Input: part model. Units: mm. Frame: model coordinates. A direction names the side the tool comes from. Round coordinates to 2 decimals unless told otherwise and drop trailing zeros. Loops run counter-clockwise (first coordinate to the right, second up) from the corner with the lowest first, then second, coordinate; pieces in that order, holes last. Notation, with made-up numbers: (81, 72) -> (135, 72) arc R10 cw to (135, 90) -> close; hole circle Ø7 at (-12.75, -25). An arc over 180 degrees is marked (long way). One line per question, with ' | ' between items. Start each with the question number.
Q1. Cut plane B-B on x = 3.5. Return loops of the section in (y, z).
Q2. Access query for faces 1 (the face through (22, 70, -15)), 2 (the face through (-8.14, 69.25, -46.06)). Directions: +Z, -Z, +X, -X, +Y, -Y. A direction counts if a zero-diameter tool reaches every point of the face in a straight line with its end or side. Return the directions, or none.
Q3. Contact query for flat-ended pins moving along their axis: P1, Ø8, axis at x = -9, y = 36, coming from the +Z side; P2, Ø2.5, axis at y = 71, z = -15, coming from the -X side; P3, Ø10, axis at y = 75.5, z = -7.5, coming from the -X side; P4, Ø10, axis at x = -20, y = 36, coming from the -Z side. Output: stop coordinate, or through.
Q4. Mould query, pull axis X, two halves, no side actions, for faces 3 (the face through (23, 54, -25)), 4 (the face through (21.028, 53.072, -3.464)), 5 (the face through (6.58, 65.9, -46.06)). Classes: pulls with the +X half, pulls with the -X half, needs draft (parallel to the pull), parting line crosses it, or undercut.
Q5. Cut plane C-C on y = 13.75. Return loops of the section in (x, z), and give its area (3 significant figures).
Q6. Cut plane D-D on z = -43.5. Return loops of the section in (x, y), and give its area (3 significant figures).
Q7. Material intervals for L1, parallel to Y at x = 22.7, z = -30.75; L2, parallel to Z at x = 22.6, y = 71; L3, parallel to Y at x = 22, z = -12, sorted ascending.
Q8. Cut plane A-A on z = -12. State how many separate pieces and enclosed holes the cut face has, and give its area (3 significant figures).
from build123d import *

# Parameters (mm, degrees)
BOSS_EXTRUDE1_DEPTH = 90
SKETCH2_R           = 10.1
CUT_EXTRUDE1_DEPTH  = 2.8
SKETCH3_R           = 2.5
SKETCH3_R_2         = 1
CUT_EXTRUDE2_DEPTH  = 22
SKETCH4_R           = 10.1
CUT_EXTRUDE3_DEPTH  = 10
FILLET1_R           = 10
CUT_EXTRUDE9_DEPTH  = 70
FILLET2_R           = 30
SKETCH9_R           = 2.5
SKETCH9_R_2         = 1
CUT_EXTRUDE11_DEPTH = 22.8
SKETCH10_R          = 10.1
CUT_EXTRUDE12_DEPTH = 2.8
SKETCH11_R          = 10.1
CUT_EXTRUDE13_DEPTH = 12.8
FILLET4_R           = 10
SKETCH13_W          = 1
SKETCH13_H          = 35
CUT_EXTRUDE14_DEPTH = 50
CUT_EXTRUDE20_DEPTH = 20


with BuildPart() as part:
    # Sketch1 → Boss-Extrude1 (new body)
    with BuildSketch(Plane(origin=(0, 0, 0), x_dir=(1, 0, 0), z_dir=(0, 1, 0))):
        Polygon((-27.5, 0), (-27.5, 42), (19, 42), (19, 0), (23, 0), (23, 50), (-30.5, 50), (-30.5, 0), align=None)
    extrude(amount=BOSS_EXTRUDE1_DEPTH)

    # Sketch2 → Cut-Extrude1 (cut)
    with BuildSketch(Plane.ZY.offset(-19)):
        with Locations((-12, 78)):
            Circle(SKETCH2_R)
    extrude(amount=-CUT_EXTRUDE1_DEPTH, mode=Mode.SUBTRACT)

    # Sketch3 → Cut-Extrude2 (cut)
    with BuildSketch(Plane.ZY.offset(-21.8)):
        with Locations((-12, 78)):
            Circle(SKETCH3_R)
        with Locations((-15, 85)):
            Circle(SKETCH3_R_2)
        with Locations((-12, 85)):
            Circle(SKETCH3_R_2)
        with Locations((-9, 85)):
            Circle(SKETCH3_R_2)
        with Locations((-19, 81)):
            Circle(SKETCH3_R_2)
        with Locations((-19, 78)):
            Circle(SKETCH3_R_2)
        with Locations((-19, 75)):
            Circle(SKETCH3_R_2)
        with Locations((-15, 71)):
            Circle(SKETCH3_R_2)
        with Locations((-12, 71)):
            Circle(SKETCH3_R_2)
        with Locations((-9, 71)):
            Circle(SKETCH3_R_2)
        with Locations((-5, 75)):
            Circle(SKETCH3_R_2)
        with Locations((-5, 78)):
            Circle(SKETCH3_R_2)
        with Locations((-5, 81)):
            Circle(SKETCH3_R_2)
    extrude(amount=-CUT_EXTRUDE2_DEPTH, mode=Mode.SUBTRACT)

    # Sketch4 → Cut-Extrude3 (cut)
    with BuildSketch(Plane.ZY.offset(30.5)):
        with Locations((-12, 78)):
            Circle(SKETCH4_R)
    extrude(amount=-CUT_EXTRUDE3_DEPTH, mode=Mode.SUBTRACT)

    # Fillet1
    fillet1_edges = [part.edges().sort_by_distance(p)[0] for p in [
        (21, 90, 0),
        (-29, 90, 0),
    ]]
    fillet(fillet1_edges, radius=FILLET1_R)

    # Sketch8 → Cut-Extrude9 (cut)
    with BuildSketch(Plane(origin=(23, 0, 0), x_dir=(0, 0, -1), z_dir=(1, 0, 0))):
        Polygon((0, 0), (10, 0), (10, 40), (0, 60), align=None)
        with BuildLine():
            Line((50, 45), (49.384007447, 45))
            ThreePointArc((49.384007447, 45), (46.548633561, 44.118331571), (44.713203531, 41.784261971))
            ThreePointArc((44.713203531, 41.784261971), (39.074197476, 21.242984276), (37.5, 0))
            Line((37.5, 0), (50, 0))
            Line((50, 0), (50, 45))
        make_face()
    extrude(amount=-CUT_EXTRUDE9_DEPTH, mode=Mode.SUBTRACT)

    # Fillet2
    fillet2_edges = [part.edges().sort_by_distance(p)[0] for p in [
        (-29, 40, -10),
        (21, 40, -10),
    ]]
    fillet(fillet2_edges, radius=FILLET2_R)

    # Sketch9 → Cut-Extrude11 (cut)
    with BuildSketch(Plane.ZY.offset(-19)):
        with Locations((-23.75, 13.75)):
            Circle(SKETCH9_R)
        with Locations((-23.75, 20.75)):
            Circle(SKETCH9_R_2)
        with Locations((-26.75, 20.75)):
            Circle(SKETCH9_R_2)
        with Locations((-20.75, 20.75)):
            Circle(SKETCH9_R_2)
        with Locations((-16.75, 10.75)):
            Circle(SKETCH9_R_2)
        with Locations((-16.75, 13.75)):
            Circle(SKETCH9_R_2)
        with Locations((-16.75, 16.75)):
            Circle(SKETCH9_R_2)
        with Locations((-26.75, 6.75)):
            Circle(SKETCH9_R_2)
        with Locations((-23.75, 6.75)):
            Circle(SKETCH9_R_2)
        with Locations((-20.75, 6.75)):
            Circle(SKETCH9_R_2)
        with Locations((-30.75, 16.75)):
            Circle(SKETCH9_R_2)
        with Locations((-30.75, 13.75)):
            Circle(SKETCH9_R_2)
        with Locations((-30.75, 10.75)):
            Circle(SKETCH9_R_2)
    extrude(amount=-CUT_EXTRUDE11_DEPTH, mode=Mode.SUBTRACT)

    # Sketch10 → Cut-Extrude12 (cut)
    with BuildSketch(Plane.ZY.offset(-19)):
        with Locations((-23.75, 13.75)):
            Circle(SKETCH10_R)
    extrude(amount=-CUT_EXTRUDE12_DEPTH, mode=Mode.SUBTRACT)

    # Sketch11 → Cut-Extrude13 (cut)
    with BuildSketch(Plane.ZY.offset(30.5)):
        with Locations((-23.75, 13.75)):
            Circle(SKETCH11_R)
    extrude(amount=-CUT_EXTRUDE13_DEPTH, mode=Mode.SUBTRACT)

    # Fillet4
    fillet4_edges = [part.edges().sort_by_distance(p)[0] for p in [
        (-29, 0, -10),
        (21, 0, -10),
        (21, 0, -37.5),
        (-29, 0, -37.5),
    ]]
    fillet(fillet4_edges, radius=FILLET4_R)

    # Sketch13 → Cut-Extrude14 (cut)
    with BuildSketch(Plane.XY):
        with Locations((-28, 17.5)):
            Rectangle(SKETCH13_W, SKETCH13_H)
    extrude(amount=-CUT_EXTRUDE14_DEPTH, mode=Mode.SUBTRACT)

    # Sketch14 → Cut-Extrude20 (cut)
    with BuildSketch(Plane(origin=(0, 0, -50), x_dir=(-1, 0, 0), z_dir=(0, 0, -1))):
        with BuildLine():
            Line((3.27778227, 69.250932504), (2.845176463, 68.801688012))
            ThreePointArc((2.845176463, 68.801688012), (0.391852409, 70.892666632), (-2.246261107, 72.745056327))
            ThreePointArc((-2.246261107, 72.745056327), (-6.625047437, 65.79780173), (-8.487956293, 57.799821563))
            ThreePointArc((-8.487956293, 57.799821563), (-5.961417112, 64.793099841), (-1.768021606, 70.933521279))
            ThreePointArc((-1.768021606, 70.933521279), (0.045073944, 69.272193574), (1.971595392, 67.743847957))
            ThreePointArc((1.971595392, 67.743847957), (-1.648113464, 59.360569649), (-0.654011446, 50.283488148))
            ThreePointArc((-0.654011446, 50.283488148), (-0.301953995, 59.840560068), (4.104319798, 68.328570399))
            ThreePointArc((4.104319798, 68.328570399), (8.510593592, 59.840560068), (8.862651043, 50.283488148))
            ThreePointArc((8.862651043, 50.283488148), (9.856753061, 59.360569649), (6.237044205, 67.743847957))
            ThreePointArc((6.237044205, 67.743847957), (8.163565653, 69.272193574), (9.976661203, 70.933521279))
            ThreePointArc((9.976661203, 70.933521279), (14.170056709, 64.793099841), (16.69659589, 57.799821563))
            ThreePointArc((16.69659589, 57.799821563), (14.833687034, 65.79780173), (10.454900704, 72.745056327))
            ThreePointArc((10.454900704, 72.745056327), (7.816787188, 70.892666632), (5.363463133, 68.801688012))
            Line((5.363463133, 68.801688012), (4.930857327, 69.250932504))
            ThreePointArc((4.930857327, 69.250932504), (7.415465307, 71.667758801), (10.199165492, 73.733028626))
            ThreePointArc((10.199165492, 73.733028626), (9.57768596, 80.703606058), (7.041999649, 87.2262958))
            ThreePointArc((7.041999649, 87.2262958), (8.295873303, 80.714857968), (8.669787468, 74.094343639))
            ThreePointArc((8.669787468, 74.094343639), (6.272067499, 72.3318465), (4.104319798, 70.29313928))
            ThreePointArc((4.104319798, 70.29313928), (1.936572098, 72.3318465), (-0.461147871, 74.094343639))
            ThreePointArc((-0.461147871, 74.094343639), (-0.087233707, 80.714857968), (1.166639948, 87.2262958))
            ThreePointArc((1.166639948, 87.2262958), (-1.369046364, 80.703606058), (-1.990525895, 73.733028626))
            ThreePointArc((-1.990525895, 73.733028626), (0.79317429, 71.667758801), (3.27778227, 69.250932504))
        make_face()
    extrude(amount=-CUT_EXTRUDE20_DEPTH, mode=Mode.SUBTRACT)


solid = part.part
Results:
1) outline: (33.77, -42) arc R110 cw to (41.78, -44.71) arc R5 cw to (45, -49.38) -> (45, -50) -> (68.79, -50) -> (68.79, -42) -> close; (71.22, -50) -> (90, -50) -> (90, -42) -> (71.22, -42) -> close
2) face 1: +X, -X | face 2: +Z, -Z
3) P1: z = -42 | P2: x = 21.8 | P3: x = -30.5 | P4: z = -44.42
4) face 3: pulls with the +X half | face 4: needs draft | face 5: undercut
5) outline: (-30.5, -38.04) -> (-28.5, -38.04) -> (-28.5, -33.85) -> (-30.5, -33.85) -> close; (-30.5, -13.65) -> (-28.5, -13.65) -> (-28.5, -10) -> (-30.5, -10) -> close; (19, -38.04) -> (23, -38.04) -> (23, -31.75) -> (21.8, -31.75) -> (21.8, -33.85) -> (19, -33.85) -> close; (19, -13.65) -> (21.8, -13.65) -> (21.8, -15.75) -> (23, -15.75) -> (23, -10) -> (19, -10) -> close; (21.8, -29.75) -> (23, -29.75) -> (23, -26.25) -> (21.8, -26.25) -> close; (21.8, -21.25) -> (23, -21.25) -> (23, -17.75) -> (21.8, -17.75) -> close | area: 60.5 mm^2
6) outline: (-30.5, 38.45) -> (23, 38.45) -> (23, 90) -> (-30.5, 90) -> close; hole (-16.7, 57.8) arc R29.53 cw to (-9.98, 70.93) arc R34.6 ccw to (-6.24, 67.74) arc R17.87 ccw to (-8.86, 50.28) arc R21.81 cw to (-4.1, 68.33) arc R21.81 cw to (0.65, 50.28) arc R17.87 ccw to (-1.97, 67.74) arc R34.6 ccw to (1.77, 70.93) arc R29.53 cw to (8.49, 57.8) arc R24.73 ccw to (2.25, 72.75) arc R34.43 ccw to (-2.85, 68.8) -> (-3.28, 69.25) arc R26.03 cw to (1.99, 73.73) arc R24.91 ccw to (-1.17, 87.23) arc R49.59 cw to (0.46, 74.09) arc R24.64 ccw to (-4.1, 70.29) arc R24.64 ccw to (-8.67, 74.09) arc R49.59 cw to (-7.04, 87.23) arc R24.91 ccw to (-10.2, 73.73) arc R26.03 cw to (-4.93, 69.25) -> (-5.36, 68.8) arc R34.43 ccw to (-10.45, 72.75) arc R24.73 ccw to start | area: 2,620 mm^2
7) L1: 0.48 to 9.75, 11.75 to 12.75, 14.75 to 15.75, 17.75 to 90 | L2: -50 to -16, -14 to -13, -11 to -10, -8 to 0 | L3: 4 to 70, 72 to 75.5, 80.5 to 84, 86 to 90
8) separate pieces: 6 | enclosed holes: 0 | area: 443 mm^2
